Here's how the part is built. I have some questions about the finished solid (model axes, mm). Face numbers are marked on the shaded views. A direction names the side the tool comes from. Coordinates: 2 decimals unless noted, no trailing zeros. Loops run counter-clockwise (first coordinate to the right, second up) from the corner with the lowest first, then second, coordinate; pieces in that order, holes last. Notation, with made-up numbers: (28.5, 11.5) -> (53.5, 11.5) arc R9 ccw to (53.5, 28.5) -> close; hole circle Ø11 at (17.5, 55.25). An arc over 180 degrees is marked (long way). Answer as a JSON object with one key per item and string values. Group by question number.
1) I'm going to push flat-ended pins straight in: pin 1 (3.5 mm diameter, centred on x = 34.89, z = -40.81, fed in from +Y); pin 2 (3.5 mm diameter, centred on x = 55.5, y = 3, fed in from +Z); pin 3 (3 mm diameter, centred on y = 17, z = 1.5, fed in from +X); pin 4 (2.5 mm diameter, centred on x = 34.89, z = -40.81, fed in from -Y) (3 decimals). Where does each tip first touch, or does it pass through?
2) I want a section at B-B (z = -26). Write out the boundary of the cut face in (x, y).
3) I want a section at C-C (z = 38). Write out the boundary of the cut face in (x, y).
4) I want a section at A-A (y = 0). Write out the boundary of the cut face in (x, z).
5) I want a section at D-D (z = 12). Write out the boundary of the cut face in (x, y), then the cut area to 3 significant figures.
6) If we mould it in two halves opening along X, with no side actions, what happens to the marked faces 4, 5 and 6? For each: +X half, -X half, draft (parallel to the pull), parting line (faces both ways), or undercut.
7) Which directions (+Z, -Z, +X, -X, +Y, -Y) give clear straight access to the entire face, cutting with the end or side of a thin tool? Please do the marked faces 1, 2 and 3.
8) I need wall thicknesses on probe 1 along Y at (x, z) = (48, -16); probe 2 along Y at (x, z) = (4, 0); probe 3 along X at (y, z) = (19, 12.5). Which ranges of each line are inside material? Lowest first, please. Write a range as [from, to].
```python
from build123d import *

# Parameters (mm, degrees)
SKETCH1_R               = 35
BOSS_EXTRUDE2_DEPTH     = 10
SKETCH3_R               = 23.5
BOSS_EXTRUDE3_DEPTH     = 15
BOSS_EXTRUDE4_DEPTH     = 4
SKETCH7_R               = 1.5
CUT_EXTRUDE1_DEPTH      = 4
MIRROR2_COPY_1_SKETCH_R = 1.5
MIRROR2_COPY_1_DEPTH    = 4
SKETCH9_W               = 4
SKETCH9_H               = 9
BOSS_EXTRUDE5_DEPTH     = 5
FILLET1_R               = 2
FILLET1_OF_MIRROR3_R    = 2
SKETCH10_W              = 14
SKETCH10_H              = 26
BOSS_EXTRUDE6_DEPTH     = 3
SKETCH11_R              = 10
CUT_EXTRUDE2_DEPTH      = 10


with BuildPart() as part:
    # Sketch1 → Boss-Extrude2 (new body)
    with BuildSketch(Plane(origin=(0, 0, 0), x_dir=(0, 0, -1), z_dir=(1, 0, 0))):
        Circle(SKETCH1_R)
    extrude(amount=BOSS_EXTRUDE2_DEPTH)

    # Sketch3 → Boss-Extrude3 (add)
    with BuildSketch(Plane(origin=(10, 0, 0), x_dir=(0, 0, -1), z_dir=(1, 0, 0))):
        Circle(SKETCH3_R)
    extrude(amount=BOSS_EXTRUDE3_DEPTH)

    # Sketch5 → Boss-Extrude4 (add)
    with BuildSketch(Plane(origin=(0, 13, 0), x_dir=(1, 0, 0), z_dir=(0, 1, 0))):
        Polygon((25, 35), (25, -35), (32.392057511, -43.809511096), (37.392057511, -43.809511096), (54.425929168, -23.509333353), (54.425929168, 23.509333353), (37.392057511, 43.809511096), (32.392057511, 43.809511096), align=None)
    boss_extrude4 = extrude(amount=-BOSS_EXTRUDE4_DEPTH)

    # Sketch7 → Cut-Extrude1 (cut)
    with BuildSketch(Plane(origin=(0, 13, 0), x_dir=(1, 0, 0), z_dir=(0, 1, 0))):
        with Locations(Location((34.892057511, -40.809511096, 0), (0, 0, 270))):
            Circle(SKETCH7_R)
    cut_extrude1 = extrude(amount=-CUT_EXTRUDE1_DEPTH, mode=Mode.SUBTRACT)

    # Mirror1: Cut-Extrude1 across plane
    add(cut_extrude1.mirror(Plane.XY), mode=Mode.SUBTRACT)

    # Mirror2: Boss-Extrude4, Cut-Extrude1 across plane
    add(boss_extrude4.mirror(Plane.ZX))
    add(cut_extrude1.mirror(Plane.ZX), mode=Mode.SUBTRACT)

    # Mirror2 copy 1 sketch → Mirror2 copy 1 (cut)
    with BuildSketch(Plane.XZ.offset(13)):
        with Locations(Location((34.892057511, -40.809511096, 0), (0, 0, 270))):
            Circle(MIRROR2_COPY_1_SKETCH_R)
    extrude(amount=-MIRROR2_COPY_1_DEPTH, mode=Mode.SUBTRACT)

    # Sketch9 → Boss-Extrude5 (add)
    with BuildSketch(Plane(origin=(25, 0, 0), x_dir=(0, 0, -1), z_dir=(1, 0, 0))):
        with Locations((0, 17.5)):
            Rectangle(SKETCH9_W, SKETCH9_H)
    boss_extrude5 = extrude(amount=BOSS_EXTRUDE5_DEPTH)

    # Fillet1
    fillet1_edges = [part.edges().sort_by_distance(p)[0] for p in [
        (27.5, 22, -2),
        (27.5, 22, 2),
    ]]
    fillet(fillet1_edges, radius=FILLET1_R - 0.0001)  # a hair under: the kernel refuses the full size

    # Mirror3: Boss-Extrude5 across plane
    add(boss_extrude5.mirror(Plane.ZX))

    # Fillet1 of Mirror3
    fillet1_of_mirror3_edges = [part.edges().sort_by_distance(p)[0] for p in [
        (27.5, -22, -2),
        (27.5, -22, 2),
    ]]
    fillet(fillet1_of_mirror3_edges, radius=FILLET1_OF_MIRROR3_R - 0.0001)  # a hair under: the kernel refuses the full size

    # Sketch10 → Boss-Extrude6 (add)
    with BuildSketch(Plane(origin=(54.425929168, 0, 0), x_dir=(0, 0, -1), z_dir=(1, 0, 0))):
        Rectangle(SKETCH10_W, SKETCH10_H)
    extrude(amount=BOSS_EXTRUDE6_DEPTH)

    # Sketch11 → Cut-Extrude2 (cut)
    with BuildSketch(Plane.ZY):
        Circle(SKETCH11_R)
    extrude(amount=-CUT_EXTRUDE2_DEPTH, mode=Mode.SUBTRACT)


solid = part.part
```
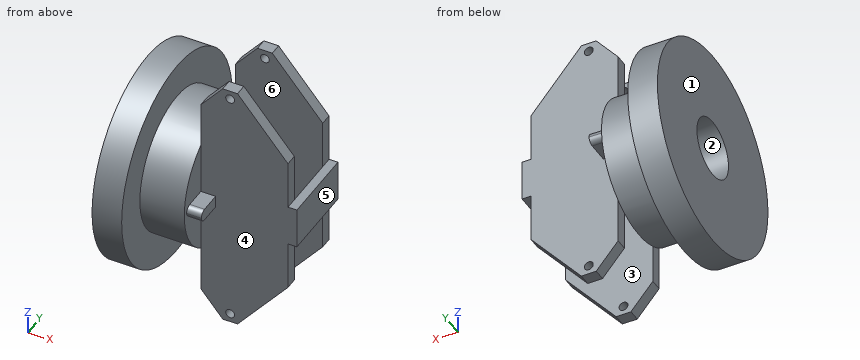
Determined:
{
 "1": {"pin 1": "y = 13", "pin 2": "z = 7", "pin 3": "x = 30", "pin 4": "through"},
 "2": {"outline": "(0, -23.43) -> (10, -23.43) -> (10, 23.43) -> (0, 23.43) -> close; (25, -13) -> (52.34, -13) -> (52.34, -9) -> (25, -9) -> close; (25, 9) -> (52.34, 9) -> (52.34, 13) -> (25, 13) -> close"},
 "3": {"outline": "(27.52, -13) -> (42.27, -13) -> (42.27, -9) -> (27.52, -9) -> close; (27.52, 9) -> (42.27, 9) -> (42.27, 13) -> (27.52, 13) -> close"},
 "4": {"outline": "(0, -35) -> (10, -35) -> (10, -23.5) -> (25, -23.5) -> (25, 23.5) -> (10, 23.5) -> (10, 35) -> (0, 35) -> (0, 10) -> (10, 10) -> (10, -10) -> (0, -10) -> close; (54.43, -7) -> (57.43, -7) -> (57.43, 7) -> (54.43, 7) -> close"},
 "5": {"outline": "(0, -32.88) -> (10, -32.88) -> (10, -20.21) -> (25, -20.21) -> (25, -13) -> (54.43, -13) -> (54.43, -9) -> (25, -9) -> (25, 9) -> (54.43, 9) -> (54.43, 13) -> (25, 13) -> (25, 20.21) -> (10, 20.21) -> (10, 32.88) -> (0, 32.88) -> close", "area": "1,500 mm^2"},
 "6": {"face 4": "draft", "face 5": "+X half", "face 6": "undercut"},
 "7": {"face 1": "+Z, -Z, -X, +Y, -Y", "face 2": "-X", "face 3": "+Z, -Z"},
 "8": {"probe 1": "[-13, -9], [9, 13]", "probe 2": "[-35, -10], [10, 35]", "probe 3": "[0, 25]"}
}
